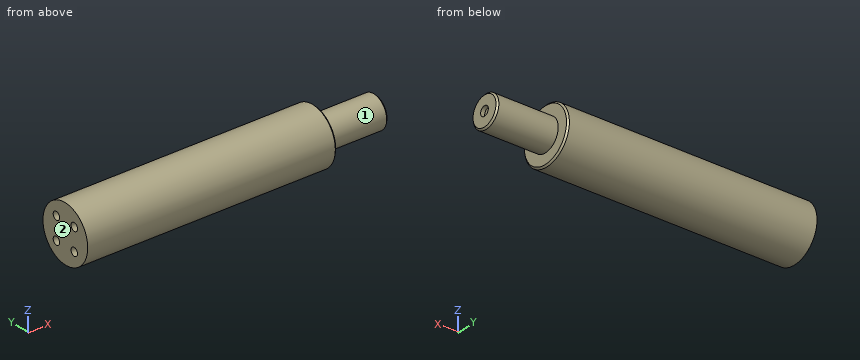
from build123d import *

# Parameters (mm, degrees)
CHAMFER1_SIZE      = 1
SKETCH2_R          = 2.5
CUT_EXTRUDE1_DEPTH = 27


with BuildPart() as part:
    # Sketch1 → Revolve1 (revolve)
    with BuildSketch(Plane.XY, mode=Mode.PRIVATE) as revolve1_sk:
        Polygon((190.9, 0), (190.9, 3), (193.4, 3), (193.4, 10), (155.4, 10), (155.4, 17.5), (0, 17.5), (0, 0), align=None)
    revolve(revolve1_sk.sketch.rotate(Axis((0, 0, 0), (1, 0, 0)), 90), axis=Axis((0, 0, 0), (1, 0, 0)))

    # Chamfer1
    chamfer1_edges = [part.edges().sort_by_distance(p)[0] for p in [
        (193.4, 0, -10),
        (155.4, 0, -17.5),
    ]]
    chamfer(chamfer1_edges, length=CHAMFER1_SIZE)

    # Sketch2 → Cut-Extrude1 (cut)
    with BuildSketch(Plane.ZY):
        with Locations((-7, 7)):
            Circle(SKETCH2_R)
        with Locations(Location((7, 7, 0), (0, 0, 180))):
            Circle(SKETCH2_R)
        with Locations((7, -7)):
            Circle(SKETCH2_R)
        with Locations(Location((-7, -7, 0), (0, 0, 180))):
            Circle(SKETCH2_R)
    extrude(amount=-CUT_EXTRUDE1_DEPTH, mode=Mode.SUBTRACT)


solid = part.part
Part model, mm, in its own coordinate system. Face numbers are marked on the shaded views. A direction names the side the tool comes from. Coordinates: 2 decimals unless noted, no trailing zeros. Loops run counter-clockwise (first coordinate to the right, second up) from the corner with the lowest first, then second, coordinate; pieces in that order, holes last. Notation, with made-up numbers: (69, 31.25) -> (97, 31.25) arc R10 ccw to (97, 43.25) -> close; hole circle Ø7 at (-10, -25). An arc over 180 degrees is marked (long way). Use a Markdown table: item, result. Add a question column.
Item 1: Band-saw the part on D-D on x = 160.5. Write the cut outline in (y, z).
Item 2: Which spindle directions (+Z, -Z, +X, -X, +Y, -Y) get a long thin tool onto all of the face, cutting with end or side? Do the marked faces 1 and 2. Say none if no direction does.
Item 3: Band-saw the part on C-C on x = 93. Write the cut outline in (y, z).
Item 4: Probe probe 1 along Y at (x, z) = (24, 6.5); probe 2 along Y at (x, z) = (191, 0); probe 3 along Z at (x, y) = (25.5, -0.5). List the from-to ranges inside material, lowest first.
Item 5: Band-saw the part on A-A on y = 0. Write the cut outline in (x, z), plus the area to 3 significant figures.
Item 6: Flat gauge pins, fed straight in: P1, Ø5, axis at y = 0, z = 0, coming from the +X side; P2, Ø1.5, axis at y = 6.5, z = -8, coming from the -X side; P3, Ø2, axis at x = 101.5, y = -13.5, coming from the +Z side. Where does each tip first touch, or does it go through?
Geometry says:
| question | item | result |
|---|---|---|
| 1 | outline | circle Ø20 at (0, 0) |
| 2 | face 1 | +X |
| 2 | face 2 | +Z, -Z, -X, +Y, -Y |
| 3 | outline | circle Ø35 at (0, 0) |
| 4 | probe 1 | -16.25 to -9.45, -4.55 to 4.55, 9.45 to 16.25 |
| 4 | probe 2 | -10 to -3, 3 to 10 |
| 4 | probe 3 | -17.49 to 17.49 |
| 5 | outline | (0, -17.5) -> (154.4, -17.5) -> (155.4, -16.5) -> (155.4, -10) -> (192.4, -10) -> (193.4, -9) -> (193.4, -3) -> (190.9, -3) -> (190.9, 3) -> (193.4, 3) -> (193.4, 9) -> (192.4, 10) -> (155.4, 10) -> (155.4, 16.5) -> (154.4, 17.5) -> (0, 17.5) -> close |
| 5 | area | 6,180 mm² |
| 6 | P1 | x = 190.9 |
| 6 | P2 | x = 27 |
| 6 | P3 | z = 12.25 |
